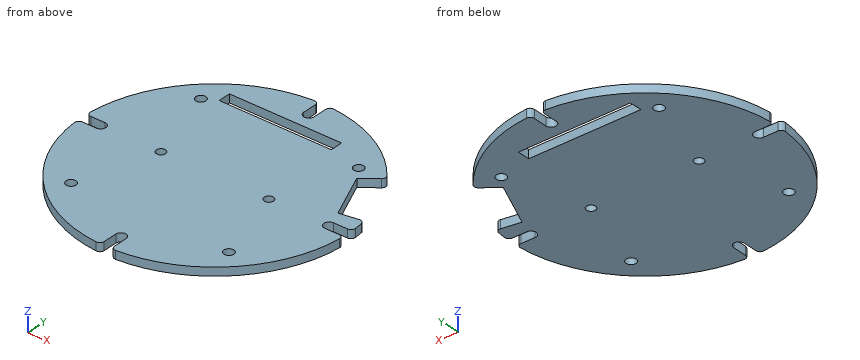
from build123d import *

# Parameters (mm, degrees)
SKETCH_1_R             = 32
EXTRUDE_1_DEPTH        = 2
SKETCH_2_R             = 1.1
CUT_EXTRUDE_1_DEPTH    = 46.299006612
HOLE_WIZARD_M2_1_D     = 2.4
HOLE_WIZARD_M2_1_DEPTH = 3.5
HOLE_WIZARD_M2_1_TIP   = 0.721032743
SKETCH_6_R             = 1.1
SKETCH_6_W             = 27
SKETCH_6_H             = 3
CUT_EXTRUDE_2_DEPTH    = 46.264500439
CUT_EXTRUDE1_DEPTH     = 10
FILLET2_R              = 1


with BuildPart() as part:
    # 스케치1 → 보스-돌출1 (new body)
    with BuildSketch(Plane.XY):
        Circle(SKETCH_1_R)
    extrude(amount=EXTRUDE_1_DEPTH)

    # 스케치2 → 컷-돌출1 (cut, through all)
    with BuildSketch(Plane.XY.offset(2)):
        with Locations((-13, 0)):
            Circle(SKETCH_2_R)
        with Locations((13, 0)):
            Circle(SKETCH_2_R)
        with BuildLine():
            Line((1.25, -27.5), (1.25, -31.975576617))
            ThreePointArc((1.25, -31.975576617), (0, -33.225576617), (-1.25, -31.975576617))
            Line((-1.25, -31.975576617), (-1.25, -27.5))
            ThreePointArc((-1.25, -27.5), (0, -26.25), (1.25, -27.5))
        make_face()
        with BuildLine():
            Line((27.5, 1.25), (32, 1.25))
            ThreePointArc((32, 1.25), (33.25, 0), (32, -1.25))
            Line((32, -1.25), (27.5, -1.25))
            ThreePointArc((27.5, -1.25), (26.25, 0), (27.5, 1.25))
        make_face()
        with BuildLine():
            Line((-27.5, -1.25), (-32, -1.25))
            ThreePointArc((-32, -1.25), (-33.25, 0), (-32, 1.25))
            Line((-32, 1.25), (-27.5, 1.25))
            ThreePointArc((-27.5, 1.25), (-26.25, 0), (-27.5, -1.25))
        make_face()
        with BuildLine():
            Line((-1.25, 27.5), (-1.25, 32))
            ThreePointArc((-1.25, 32), (0, 33.25), (1.25, 32))
            Line((1.25, 32), (1.25, 27.5))
            ThreePointArc((1.25, 27.5), (0, 26.25), (-1.25, 27.5))
        make_face()
    extrude(amount=-CUT_EXTRUDE_1_DEPTH, mode=Mode.SUBTRACT)

    # M2 여유 구멍1
    with Locations(Plane(origin=(-19, 19, 2), x_dir=(1, 0, 0), z_dir=(0, 0, 1))):
        with Locations((0, 0), (38, 0), (38, -38), (0, -38)):
            Hole(HOLE_WIZARD_M2_1_D / 2, depth=HOLE_WIZARD_M2_1_DEPTH)
            with Locations((0, 0, -(HOLE_WIZARD_M2_1_DEPTH + HOLE_WIZARD_M2_1_TIP / 2))):  # 118° drill point
                Cone(0, HOLE_WIZARD_M2_1_D / 2, HOLE_WIZARD_M2_1_TIP, mode=Mode.SUBTRACT)

    # 스케치6 → 컷-돌출2 (cut, through all)
    with BuildSketch(Plane.XY.offset(2)):
        with Locations((25, 22.2)):
            Circle(SKETCH_6_R)
        with Locations((-2.5, 22.2)):
            Rectangle(SKETCH_6_W, SKETCH_6_H)
    extrude(amount=-CUT_EXTRUDE_2_DEPTH, mode=Mode.SUBTRACT)

    # Sketch1 → Cut-Extrude1 (cut)
    with BuildSketch(Plane.XY.offset(2)):
        Polygon((21, 16), (30.255253107, 23.051621415), (39.765804764, 6.729597729), (26, 4.4), align=None)
    extrude(amount=-CUT_EXTRUDE1_DEPTH, mode=Mode.SUBTRACT)

    # Fillet2
    fillet2_edges = [part.edges().sort_by_distance(p)[0] for p in [
        (25.453815041, 19.393382888, 1),
        (31.551388335, 5.339465718, 1),
        (1.25, -31.975576617, 1),
        (-1.25, -31.975576617, 1),
        (31.975576617, 1.25, 1),
        (31.975576617, -1.25, 1),
        (-31.975576617, -1.25, 1),
        (-31.975576617, 1.25, 1),
        (-1.25, 31.975576617, 1),
        (1.25, 31.975576617, 1),
    ]]
    fillet(fillet2_edges, radius=FILLET2_R)


solid = part.part
Check sheet for the modelled part. Datum: model origin and axes. Units: mm. Round coordinates to 2 decimals unless told otherwise and drop trailing zeros. Write each loop counter-clockwise with the first axis right and the second up, starting at its lowest first coordinate (ties: lowest second). Pieces come first, ordered by that corner, then holes. Notation, with made-up numbers: (84.5, 86) - (137.5, 86) arc R33 cw to (137.5, 122) - close; hole circle Ø1 at (81, -36). An arc over 180 degrees is marked (long way). Return JSON: item names as keys, results as strings.
Q1. Scan lines: L1, parallel to Y at x = 19, z = 0.4; L2, parallel to Y at x = -13, z = 1.3; L3, parallel to X at y = 18, z = 0.6 (3 decimals). Record each from-to range of solid material in increasing order. Write a range as from..to.
Returned:
{"L1": "y = -25.75..-20.2, -17.8..17.8, 20.2..25.75", "L2": "y = -29.24..-1.1, 1.1..20.7, 23.7..29.24", "L3": "x = -26.458..-19.663, -18.337..18.337, 19.663..23.625"}
Q2. Cross-section at B-B (x = -19). Record the boundary of the cut face in (y, z), then the cut area to 3 significant figures.
Returned:
{"outline": "(-25.75, 0) - (-20.2, 0) - (-20.2, 2) - (-25.75, 2) - close; (-17.8, 0) - (17.8, 0) - (17.8, 2) - (-17.8, 2) - close; (20.2, 0) - (25.75, 0) - (25.75, 2) - (20.2, 2) - close", "area": "93.4 mm²"}
Q3. Cross-section at D-D (y = 11.5). Record the boundary of the cut face in (x, z), then the cut area to 3 significant figures.
Returned:
{"outline": "(-29.86, 0) - (22.94, 0) - (22.94, 2) - (-29.86, 2) - close", "area": "106 mm²"}
Q4. Depth check by flat-ended pin: P1, Ø1, axis at y = -28.5, z = 0.5, coming from the +X side; P2, Ø6, axis at x = 10.5, y = 24.5, coming from the -Z side; P3, Ø0.6, axis at y = -29, z = 1.5, coming from the -X side; P4, Ø0.6, axis at y = 29.5, z = 1.5, coming from the -X side. Enter the tip coordinate at first touch or a pass-through.
Returned:
{"P1": "stops at x = 15.49", "P2": "stops at z = 0", "P3": "stops at x = -14.15", "P4": "stops at x = -13.09"}
Q5. Cross-section at C-C (z = 1.05). Give the number of separate pieces and of enclosed holes in the cut face, then the cut area to 3 significant figures.
Returned:
{"separate pieces": "1", "enclosed holes": "7", "area": "2,970 mm²"}
Q6. Cross-section at A-A (x = 0). Record the boundary of the cut face in (y, z).
Returned:
{"outline": "(-26.25, 0) - (20.7, 0) - (20.7, 2) - (-26.25, 2) - close; (23.7, 0) - (26.25, 0) - (26.25, 2) - (23.7, 2) - close"}
